Verification items for the finished model (mm, model axes). Round coordinates to 2 decimals unless told otherwise and drop trailing zeros. Order: outer loops, then holes, each group sorted by start corner. A loop starts at its lowest first (then second) coordinate and runs counter-clockwise, first axis right, second up. Notation, with made-up numbers: (-4.75, -8.5) -> (5.25, -8.5) arc R18 cw to (5.25, 4.5) -> close; hole circle Ø2 at (-14.75, 32). An arc over 180 degrees is marked (long way). Write item = value, one per line. Start each with the question number.
from build123d import *

# Parameters (mm, degrees)
SKETCH1_W                     = 660.4
SKETCH1_H                     = 840.74
BOSS_EXTRUDE1_DEPTH           = 1.2192
F_8_CLEARANCE_HOLE1_D         = 4.4958
SKETCH5_W                     = 482.6
SKETCH5_H                     = 330.2
CUT_EXTRUDE1_DEPTH            = 2.54
TAP_DRILL_FOR_8_32_TAP1_D     = 3.4544
TAP_DRILL_FOR_8_32_TAP1_DEPTH = 25.4
TAP_DRILL_FOR_8_32_TAP1_TIP   = 1.037806461


with BuildPart() as part:
    # Sketch1 → Boss-Extrude1 (new body)
    with BuildSketch(Plane.XY):
        with Locations((330.2, 420.37)):
            Rectangle(SKETCH1_W, SKETCH1_H)
    extrude(amount=BOSS_EXTRUDE1_DEPTH)

    # #8 Clearance Hole1 (through all)
    with Locations(Plane.XY.offset(1.2192)):
        with Locations((25.4, 815.34), (330.2, 815.34), (635, 815.34), (25.4, 421.64), (25.4, 27.94), (635, 27.94), (635, 421.64)):
            Hole(F_8_CLEARANCE_HOLE1_D / 2)

    # Sketch5 → Cut-Extrude1 (cut)
    with BuildSketch(Plane.XY.offset(1.2192)):
        with Locations((330.2, 574.04)):
            Rectangle(SKETCH5_W, SKETCH5_H)
    extrude(amount=-CUT_EXTRUDE1_DEPTH, mode=Mode.SUBTRACT)

    # Tap Drill for #8-32 Tap1
    with Locations(Plane.XY.offset(1.2192)):
        with Locations((76.2, 751.84), (330.2, 751.84), (584.2, 751.84), (584.2, 396.24), (330.2, 396.24), (76.2, 396.24)):
            Hole(TAP_DRILL_FOR_8_32_TAP1_D / 2, depth=TAP_DRILL_FOR_8_32_TAP1_DEPTH)
            with Locations((0, 0, -(TAP_DRILL_FOR_8_32_TAP1_DEPTH + TAP_DRILL_FOR_8_32_TAP1_TIP / 2))):  # 118° drill point
                Cone(0, TAP_DRILL_FOR_8_32_TAP1_D / 2, TAP_DRILL_FOR_8_32_TAP1_TIP, mode=Mode.SUBTRACT)


solid = part.part
(1) Depth check by flat-ended pin: pin 1 (2.5 mm diameter, centred on x = 25.4, y = 815.34, fed in from +Z). Enter the tip coordinate at first touch or a pass-through.
(2) Cross-section at C-C (z = 0.65). Give the number of separate pieces and of enclosed holes in the cut face, and give its area (3 significant figures).
(3) Cross-section at B-B (x = 372). Enter the section's corners in (y, z).
(4) Scan lines: line 1 along X through (y, z) = (815.34, 0.5); line 2 along X through (y, z) = (397, 1); line 3 along Y through (x, z) = (584.2, 0.7). Record each from-to range of solid material in increasing order. Write a range as from..to.
(5) Cross-section at A-A (y = 574). Enter the section's corners in (x, z), and give its area (3 significant figures).
Outcome:
q1.pin_1 = through
q2.separate_pieces = 1
q2.enclosed_holes = 14
q2.area = 396,000 mm^2
q3.outline = (0, 0) -> (408.94, 0) -> (408.94, 1.22) -> (0, 1.22) -> close; (739.14, 0) -> (840.74, 0) -> (840.74, 1.22) -> (739.14, 1.22) -> close
q4.line_1 = 0..23.15, 27.65..327.95, 332.45..632.75, 637.25..660.4
q4.line_2 = 0..74.65, 77.75..328.65, 331.75..582.65, 585.75..660.4
q4.line_3 = 0..394.51, 397.97..750.11, 753.57..840.74
q5.outline = (0, 0) -> (88.9, 0) -> (88.9, 1.22) -> (0, 1.22) -> close; (571.5, 0) -> (660.4, 0) -> (660.4, 1.22) -> (571.5, 1.22) -> close
q5.area = 217 mm^2
